Design review of the part built by this model. Coordinates are the model's own, in mm. A direction names the side the tool comes from. Round coordinates to 2 decimals unless told otherwise and drop trailing zeros. Order: outer loops, then holes, each group sorted by start corner. A loop starts at its lowest first (then second) coordinate and runs counter-clockwise, first axis right, second up. Notation, with made-up numbers: (38, -29.5) - (43, -29.5) arc R33 ccw to (43, 0.5) - close; hole circle Ø1 at (54, -19). An arc over 180 degrees is marked (long way). Write item = value, one per line.
Autodesk Fusion 360 part; units mm, degrees
sketch "スケッチ1" plane through (0, 0, 0) normal (0, 0, 1) x (1, 0, 0) in component "GPL H200 to H150G1"
  line L0 (-21.5, 91) -> (-68.5, 91)
  line L1 (-68.5, 91) -> (-68.5, -91)
  line L2 (-68.5, -91) -> (-21.5, -91)
  line L3 (68.5, -50) -> (68.5, 80)
  line L4 (60.2198, 80) -> (-68.5, -91) construction
  line L5 (-68.5, 91) -> (45.5182, -60.4695) construction
  line L6 (-21.5, 91) -> (-21.5, 80)
  line L7 (-21.5, 80) -> (68.5, 80)
  line L8 (-68.5, -91) -> (-21.5, -91) construction
  line L9 (68.5, -50) -> (-21.5, -91)
  dimension "d14_1" = 18
  dimension "d15_1" = 180
extrude "押し出し1" add sketch "スケッチ1" along normal blind 6 makes body 1 in component "GPL H200 to H150G1"
chamfer "面取り1" distance 15 angle 45 2 edges at (-68.5, -91, 3) (-68.5, 91, 3) on bodies 1 in component "GPL H200 to H150G1"
sketch "スケッチ2" plane through (0, 0, 6) normal (0, 0, 1) x (-1, 0, 0) in component "GPL H200 to H150G1"
  line L0 (53.5, -91) -> (68.5, -76)
  line L1 (68.5, -76) -> (68.5, 76)
  line L2 (68.5, 76) -> (53.5, 91)
  line L3 (53.5, 91) -> (21.5, 91)
  line L4 (21.5, 91) -> (-68.5, 50)
  line L5 (-68.5, 50) -> (-68.5, -80)
  line L6 (-68.5, -80) -> (21.5, -80)
  line L7 (21.5, -80) -> (21.5, -91)
  line L8 (21.5, -91) -> (53.5, -91)
  line L9 (-68.5, -80) -> (-28.5, -80) construction
  line L10 (-28.5, -80) -> (-28.5, -50) construction
  line L11 (-28.5, -50) -> (-68.5, -50) construction
  line L12 (-68.5, -50) -> (-68.5, -80) construction
  line L13 (-68.5, -50) -> (-28.5, -50) construction
  line L14 (-28.5, -50) -> (-28.5, 0) construction
  line L15 (-28.5, 0) -> (-68.5, 0) construction
  line L16 (-68.5, 0) -> (-68.5, -50) construction
  point P0 (-28.5, -50)
  point P1 (-28.5, 0)
  dimension "d10" = 40
  dimension "d11" = 30
  dimension "d12" = 40
  dimension "d13" = 50
hole "穴1" at (28.5, 50, 6) at (28.5, 0, 6) direction (0, 0, -1) diameter 18 end through all bodies 1 1 in component "GPL H200 to H150G1"
sketch "スケッチ1 (2)" plane through (0, 0, 0) normal (0, 0, 1) x (1, 0, 0) in component "Component'"
  line L0 (-21.5, 91) -> (-68.5, 91)
  line L1 (-68.5, 91) -> (-68.5, -91)
  line L2 (-68.5, -91) -> (-21.5, -91)
  line L3 (68.5, -50) -> (68.5, 80)
  line L4 (60.2198, 80) -> (-68.5, -91) construction
  line L5 (-68.5, 91) -> (45.5182, -60.4695) construction
  line L6 (-21.5, 91) -> (-21.5, 80)
  line L7 (-21.5, 80) -> (68.5, 80)
  line L8 (-68.5, -91) -> (-21.5, -91) construction
  line L9 (68.5, -50) -> (-21.5, -91)
  dimension "d2_1" = 182
  dimension "d5_1" = 47
extrude "押し出し1'" add sketch "スケッチ1 (2)" along normal blind 6 separate body makes body 2 in component "Component'"
chamfer "面取り1'" distance 15 angle 45 2 edges at (-68.5, -91, 3) (-68.5, 91, 3) on bodies 2 in component "Component'"
sketch "スケッチ2 (2)" plane through (0, 0, 6) normal (0, 0, 1) x (-1, 0, 0) in component "Component'"
  line L0 (53.5, -91) -> (68.5, -76)
  line L1 (68.5, -76) -> (68.5, 76)
  line L2 (68.5, 76) -> (53.5, 91)
  line L3 (53.5, 91) -> (21.5, 91)
  line L4 (21.5, 91) -> (-68.5, 50)
  line L5 (-68.5, 50) -> (-68.5, -80)
  line L6 (-68.5, -80) -> (21.5, -80)
  line L7 (21.5, -80) -> (21.5, -91)
  line L8 (21.5, -91) -> (53.5, -91)
  line L9 (-68.5, -80) -> (-28.5, -80) construction
  line L10 (-28.5, -80) -> (-28.5, -50) construction
  line L11 (-28.5, -50) -> (-68.5, -50) construction
  line L12 (-68.5, -50) -> (-68.5, -80) construction
  line L13 (-68.5, -50) -> (-28.5, -50) construction
  line L14 (-28.5, -50) -> (-28.5, 0) construction
  line L15 (-28.5, 0) -> (-68.5, 0) construction
  line L16 (-68.5, 0) -> (-68.5, -50) construction
  point P0 (-28.5, -50)
  point P1 (-28.5, 0)
  dimension "d10_1" = 40
  dimension "d11_1" = 30
  dimension "d12_1" = 40
  dimension "d13_1" = 50
hole "穴1'" at (28.5, 50, 6) at (28.5, 0, 6) direction (0, 0, -1) diameter 18 end through all bodies 2 2 in component "Component'"
copy_body "CutPasteBodies1" bodies 1 removing the originals makes body 3
equation "d5 = 15 mm + 32 mm"
equation "d5_1 = 15 mm + 32 mm"
Item 1: Take a section at B-B, the plane z = 3.25. State the section outline as (x, y) points.
Data:
outline = (-68.5, -76) - (-53.5, -91) - (-21.5, -91) - (68.5, -50) - (68.5, 80) - (-21.5, 80) - (-21.5, 91) - (-53.5, 91) - (-68.5, 76) - close; hole circle Ø18 at (28.5, 0); hole circle Ø18 at (28.5, 50)
Item 2: Take a section at A-A, the plane y = 0. State the section outline as (x, z) points, and give its area (3 significant figures).
Data:
outline = (-68.5, 0) - (19.5, 0) - (19.5, 6) - (-68.5, 6) - close; (37.5, 0) - (68.5, 0) - (68.5, 6) - (37.5, 6) - close
area = 714 mm2
Item 3: Take a section at C-C, the plane x = 22. State the section outline as (y, z) points.
Data:
outline = (-71.18, 0) - (-6.22, 0) - (-6.22, 6) - (-71.18, 6) - close; (6.22, 0) - (43.78, 0) - (43.78, 6) - (6.22, 6) - close; (56.22, 0) - (80, 0) - (80, 6) - (56.22, 6) - close
Item 4: Insertion check: P1, Ø1.5, axis at x = 16.5, z = 4.5, coming from the +Y side; P2, Ø1.8, axis at y = 87, z = 4.5, coming from the +X side; P3, Ø3, axis at x = 3, z = 1, coming from the -Y side. Each pin has a flat end and moves straight along its axis. Give the tip position at first contact, or say it passes through.
Data:
P1 = 80
P2 = -21.5
P3 = -80.52
Item 5: Take a section at D-D, the plane y = 46. State the section outline as (x, z) points.
Data:
outline = (-68.5, 0) - (20.44, 0) - (20.44, 6) - (-68.5, 6) - close; (36.56, 0) - (68.5, 0) - (68.5, 6) - (36.56, 6) - close
Item 6: For line 1 along X through (y, z) = (50, 4.2); line 2 along Y through (x, z) = (28.5, 2.55); line 3 along X through (y, z) = (-2.5, 2.7), list the stretches that pass through material, from the lowest coordinate up. Write a range as [from, to].
Data:
line_1 = [-68.5, 19.5], [37.5, 68.5]
line_2 = [-68.22, -9], [9, 41], [59, 80]
line_3 = [-68.5, 19.85], [37.15, 68.5]
Item 7: For faces 4 (the face through (-61.1, -83.4, 3)), 5 (the face through (23, 80, 3)), list the 3-axis set-ups (+Z, -Z, +X, -X, +Y, -Y) from which the entire face can be reached by the end or side of a thin tool; tool diameter is ignored.
Data:
face_4 = +Z, -Z, -X, -Y
face_5 = +Z, -Z, +X, +Y
Item 8: The part is to be moulded in two halves that separate along X. For faces 1 (the face through (-21.5, 86, 3)), 2 (the face through (22.417, 56.633, 2.958)), 3 (the face through (-38, -91, 3)), say which applies: +X half, -X half, draft (parallel to the pull), parting line (faces both ways), or undercut.
Data:
face_1 = +X half
face_2 = undercut
face_3 = draft
